```python
from build123d import *

# Parameters (mm, degrees)
SKETCH1_R           = 4.75
BOSS_EXTRUDE1_DEPTH = 32
SKETCH2_R           = 1.8
CUT_EXTRUDE1_DEPTH  = 3
SKETCH3_R           = 19.5
BOSS_EXTRUDE2_DEPTH = 2


with BuildPart() as part:
    # Sketch1 → Boss-Extrude1 (new body)
    with BuildSketch(Plane(origin=(0, 0, 0), x_dir=(1, 0, 0), z_dir=(0, 1, 0))):
        Circle(SKETCH1_R)
    extrude(amount=BOSS_EXTRUDE1_DEPTH)

    # Sketch2 → Cut-Extrude1 (cut)
    with BuildSketch(Plane.XZ):
        Circle(SKETCH2_R)
    extrude(amount=-CUT_EXTRUDE1_DEPTH, mode=Mode.SUBTRACT)

    # Sketch3 → Boss-Extrude2 (add)
    with BuildSketch(Plane(origin=(0, 32, 0), x_dir=(1, 0, 0), z_dir=(0, 1, 0))):
        with Locations((8.56, 4.02)):
            Circle(SKETCH3_R)
    extrude(amount=BOSS_EXTRUDE2_DEPTH)


solid = part.part
```
Design review of the part built by this model. Coordinates are the model's own, in mm. A direction names the side the tool comes from. Coordinates: 2 decimals unless noted, no trailing zeros. Loops run counter-clockwise (first coordinate to the right, second up) from the corner with the lowest first, then second, coordinate; pieces in that order, holes last. Notation, with made-up numbers: (-20, 83.25) -> (8, 83.25) arc R13 ccw to (8, 106.25) -> close; hole circle Ø3 at (-16, -9). An arc over 180 degrees is marked (long way). Answer as a JSON object with one key per item and string values.
Q1. To check wall thickness, follow L1, parallel to Y at x = -3.5, z = -14.5; L2, parallel to Z at x = 4, y = 17; L3, parallel to Z at x = -2.5, y = 14. State the ranges of each line that lie inside material, in increasing order.
Answer block:
{"L1": "y = 32 to 34", "L2": "z = -2.56 to 2.56", "L3": "z = -4.04 to 4.04"}
Q2. The part is to be moulded in two halves that separate along X. For faces 3 (the flat face through (8, 34, -4)), 4 (the flat face through (0, 3, 0)), 5 (the cylindrical face through (2.192, 15.776, 4.214)), say which applies: +X half, -X half, draft (parallel to the pull), parting line (faces both ways), or undercut.
Answer block:
{"face 3": "draft", "face 4": "undercut", "face 5": "parting line"}
Q3. Clearance check with flat-ended pins moving along their axes: pin 1 Ø2 at (y, z) = (24, 0.5) entering from -X; pin 2 Ø1 at (y, z) = (26, -3.5) entering from +X; pin 3 Ø19.5 at (x, z) = (17, -8) entering from -Y; pin 4 Ø4 at (x, z) = (0.5, 0.5) entering from -Y. State where each tip first meets the part, or that it passes through.
Answer block:
{"pin 1": "stops at x = -4.75", "pin 2": "stops at x = 3.68", "pin 3": "stops at y = 32", "pin 4": "stops at y = 0"}
Q4. Tool access review of faces 1 (the cylindrical face through (26.573, 32.986, 3.449)), 2 (the cylindrical face through (1.717, 1.479, 0.541)): name each direction out of +Z, -Z, +X, -X, +Y, -Y from which nothing blocks a thin tool from reaching the whole face with its end or side.
Answer block:
{"face 1": "+Y, -Y", "face 2": "-Y"}
Q5. Take a section at A-A on z = 0. Give the boundary of the cut face in (x, y), plus the area to 3 significant figures.
Answer block:
{"outline": "(-10.52, 32) -> (-4.75, 32) -> (-4.75, 0) -> (-1.8, 0) -> (-1.8, 3) -> (1.8, 3) -> (1.8, 0) -> (4.75, 0) -> (4.75, 32) -> (27.64, 32) -> (27.64, 34) -> (-10.52, 34) -> close", "area": "370 mm^2"}
Q6. Take a section at B-B on x = 0. Give the boundary of the cut face in (y, z).
Answer block:
{"outline": "(0, -4.75) -> (32, -4.75) -> (32, -21.54) -> (34, -21.54) -> (34, 13.5) -> (32, 13.5) -> (32, 4.75) -> (0, 4.75) -> (0, 1.8) -> (3, 1.8) -> (3, -1.8) -> (0, -1.8) -> close"}
Q7. Take a section at C-C on y = 19.5. Give the boundary of the cut face in (x, z).
Answer block:
{"outline": "circle Ø9.5 at (0, 0)"}
Q8. Take a section at D-D on x = 8.56. Give the boundary of the cut face in (y, z), plus the area to 3 significant figures.
Answer block:
{"outline": "(32, -23.52) -> (34, -23.52) -> (34, 15.48) -> (32, 15.48) -> close", "area": "78.0 mm^2"}
